```python
from build123d import *

# Parameters (mm, degrees)
F0_R     = 11.1
F1_DEPTH = 7


with BuildPart() as f1:
    # F0 (on Top) → F1 (new body)
    with BuildSketch(Plane.XY):
        with BuildLine():
            ThreePointArc((6.955402, -10.386163), (11.02707, -5.886742), (12.5, 0))
            ThreePointArc((12.5, 0), (11.02707, 5.886742), (6.955402, 10.386163))
            ThreePointArc((6.955402, 10.386163), (6.25, 10.825318), (5.51698, 11.216636))
            ThreePointArc((5.51698, 11.216636), (-6.25, 10.825318), (-12.472382, 0.830473))
            ThreePointArc((-12.472382, 0.830473), (-12.5, 0), (-12.472382, -0.830473))
            ThreePointArc((-12.472382, -0.830473), (-6.25, -10.825318), (5.51698, -11.216636))
            ThreePointArc((5.51698, -11.216636), (6.25, -10.825318), (6.955402, -10.386163))
        make_face()
        Circle(F0_R, mode=Mode.SUBTRACT)
        with BuildLine():
            ThreePointArc((6.955402, 10.386163), (11.02707, 5.886742), (12.5, 0))
            Line((12.5, 0), (14.7, 0))
            ThreePointArc((14.7, 0), (16.17293, 5.886742), (20.244598, 10.386163))
            ThreePointArc((20.244598, 10.386163), (13.6, 9.749651), (6.955402, 10.386163))
        make_face()
        with BuildLine():
            Line((14.7, 0), (12.5, 0))
            ThreePointArc((12.5, 0), (11.02707, -5.886742), (6.955402, -10.386163))
            ThreePointArc((6.955402, -10.386163), (13.6, -9.749651), (20.244598, -10.386163))
            ThreePointArc((20.244598, -10.386163), (16.17293, -5.886742), (14.7, 0))
        make_face()
        with BuildLine():
            ThreePointArc((38.3, 0), (27.2, 11.1), (16.1, 0))
            ThreePointArc((16.1, 0), (27.2, -11.1), (38.3, 0))
        make_face()
        with BuildLine():
            ThreePointArc((20.244598, 10.386163), (16.17293, 5.886742), (14.7, 0))
            ThreePointArc((14.7, 0), (16.17293, -5.886742), (20.244598, -10.386163))
            ThreePointArc((20.244598, -10.386163), (33.086742, -11.02707), (39.7, 0))
            ThreePointArc((39.7, 0), (33.086742, 11.02707), (20.244598, 10.386163))
        make_face()
        with BuildLine():
            ThreePointArc((38.3, 0), (27.2, -11.1), (16.1, 0))
            ThreePointArc((16.1, 0), (27.2, 11.1), (38.3, 0))
        make_face(mode=Mode.SUBTRACT)
        with BuildLine():
            ThreePointArc((-12.472382, 0.830473), (-6.25, 10.825318), (5.51698, 11.216636))
            ThreePointArc((5.51698, 11.216636), (1.643446, 16.652771), (-1.127618, 22.725418))
            ThreePointArc((-1.127618, 22.725418), (-7.35, 12.730573), (-19.11698, 12.339255))
            ThreePointArc((-19.11698, 12.339255), (-15.243446, 6.90312), (-12.472382, 0.830473))
        make_face()
        with BuildLine():
            ThreePointArc((-1.127618, -22.725418), (1.643446, -16.652771), (5.51698, -11.216636))
            ThreePointArc((5.51698, -11.216636), (-6.25, -10.825318), (-12.472382, -0.830473))
            ThreePointArc((-12.472382, -0.830473), (-15.243446, -6.90312), (-19.11698, -12.339255))
            ThreePointArc((-19.11698, -12.339255), (-7.35, -12.730573), (-1.127618, -22.725418))
        make_face()
        with BuildLine():
            ThreePointArc((-19.11698, 12.339255), (-7.35, 12.730573), (-1.127618, 22.725418))
            ThreePointArc((-1.127618, 22.725418), (-1.106906, 23.140425), (-1.1, 23.555891))
            ThreePointArc((-1.1, 23.555891), (-20.206351, 34.167494), (-19.11698, 12.339255))
        make_face()
        with Locations((-13.6, 23.555891)):
            Circle(F0_R, mode=Mode.SUBTRACT)
        with BuildLine():
            ThreePointArc((-1.1, -23.555891), (-1.106906, -23.140425), (-1.127618, -22.725418))
            ThreePointArc((-1.127618, -22.725418), (-7.35, -12.730573), (-19.11698, -12.339255))
            ThreePointArc((-19.11698, -12.339255), (-20.206351, -34.167494), (-1.1, -23.555891))
        make_face()
        with Locations((-13.6, -23.555891)):
            Circle(F0_R, mode=Mode.SUBTRACT)
    extrude(amount=F1_DEPTH)


solid = f1.part
```
Part model, mm, in its own coordinate system. A direction names the side the tool comes from. Coordinates: 2 decimals unless noted, no trailing zeros. Order: outer loops, then holes, each group sorted by start corner. A loop starts at its lowest first (then second) coordinate and runs counter-clockwise, first axis right, second up. Notation, with made-up numbers: (40, 74) - (82, 74) arc R34 ccw to (82, 105) - close; hole circle Ø5 at (25, 8.25). An arc over 180 degrees is marked (long way). Return JSON: item names as keys, results as strings. Group by question number.
Item 1: Cut at B-B (z = 3). List the corners of the cut face in (x, y), plus the area to 3 significant figures.
Item 2: Pin check, flat tip, straight feed: pin 1 (1.5 mm diameter, centred on x = 25.5, z = 3, fed in from +Y). Stop position of the tip, or through.
Item 3: Cut at D-D (y = 8). List the corners of the cut face in (x, z), plus the area to 3 significant figures.
Item 4: Pull direction X, two halves, no side cores. Call faces 1 (the face through (-20.519, -33.966, 3.451)), 2 (the face through (5.97, 9.36, 3.45)), 3 (the face through (-15.197, -6.822, 3.451)): pulls with the +X half, pulls with the -X half, needs draft (parallel to the pull), parting line crosses it, or undercut.
Item 5: Cut at A-A (y = -16). List the corners of the cut face in (x, z), plus the area to 3 significant figures.
Item 6: Which spindle directions (+Z, -Z, +X, -X, +Y, -Y) get a long thin tool onto all of the face, cutting with end or side? Do faces 4 (the face through (38.29, 0.49, 3.45)), 5 (the face through (-15.3, 7, 3.5)). Say none if no direction does.
Item 7: Drill centre lines: probe 1 along Y at (x, z) = (-3.5, 3.25); probe 2 along X at (y, z) = (2.5, 1); probe 3 along X at (y, z) = (-5, 6). Where is each one in solid material? Low to high. Write a range as from..to.
Item 8: Cut at C-C (x = 27.2). List the corners of the cut face in (y, z), plus the area to 3 significant figures.
Check values:
{
 "1": {"outline": "(-19.12, -12.34) arc R12.5 ccw (long way) to (-1.1, -23.56) arc R12.5 ccw to (-1.13, -22.73) arc R35 cw to (5.52, -11.22) arc R12.5 ccw to (6.96, -10.39) arc R35 cw to (20.24, -10.39) arc R12.5 ccw (long way) to (20.24, 10.39) arc R35 cw to (6.96, 10.39) arc R12.5 ccw to (5.52, 11.22) arc R35 cw to (-1.13, 22.73) arc R12.5 ccw to (-1.1, 23.56) arc R12.5 ccw (long way) to (-19.12, 12.34) arc R35 cw to (-12.47, 0.83) arc R12.5 ccw to (-12.47, -0.83) arc R35 cw to start; hole circle Ø22.2 at (-13.6, -23.56); hole circle Ø22.2 at (-13.6, 23.56); hole circle Ø22.2 at (0, 0); hole circle Ø22.2 at (27.2, 0)", "area": "723 mm2"},
 "2": {"pin 1": "stops at y = 12.46"},
 "3": {"outline": "(-15.9, 0) - (-7.69, 0) - (-7.69, 7) - (-15.9, 7) - close; (7.69, 0) - (19.51, 0) - (19.51, 7) - (7.69, 7) - close; (34.89, 0) - (36.8, 0) - (36.8, 7) - (34.89, 7) - close", "area": "154 mm2"},
 "4": {"face 1": "parting line crosses it", "face 2": "undercut", "face 3": "pulls with the -X half"},
 "5": {"outline": "(-23.56, 0) - (-21.73, 0) - (-21.73, 7) - (-23.56, 7) - close; (-5.47, 0) - (2.03, 0) - (2.03, 7) - (-5.47, 7) - close", "area": "65.3 mm2"},
 "6": {"face 4": "+Z, -Z", "face 5": "+Z, -Z, -X"},
 "7": {"probe 1": "y = -30.92..-28.16, -18.95..-10.53, 10.53..18.95, 28.16..30.92", "probe 2": "x = -13.1..-10.81, 10.81..16.39, 38.01..39.45", "probe 3": "x = -14.22..-9.91, 9.91..17.29, 37.11..38.66"},
 "8": {"outline": "(-12.5, 0) - (-11.1, 0) - (-11.1, 7) - (-12.5, 7) - close; (11.1, 0) - (12.5, 0) - (12.5, 7) - (11.1, 7) - close", "area": "19.6 mm2"}
}
